Here's how the part is built. I have some questions about the finished solid (model axes, mm). A direction names the side the tool comes from. Coordinates: 2 decimals unless noted, no trailing zeros. Write each loop counter-clockwise with the first axis right and the second up, starting at its lowest first coordinate (ties: lowest second). Pieces come first, ordered by that corner, then holes.
```python
from build123d import *

# Parameters (mm, degrees)
F1_DEPTH = 2


with BuildPart() as f1:
    # F0 (on Top) → F1 (new body)
    with BuildSketch(Plane.XY):
        Polygon((-24.640209, 27.888809), (-21.827112, 25.045134), (-37.467321, 9.5731), (-40.280418, 12.416774), (-60.897057, -7.978181), (56.897057, -7.978181), (36.280418, 12.416774), (33.467321, 9.5731), (17.827112, 25.045134), (20.640209, 27.888809), (5, 43.360843), (5, 53.360843), (-9, 53.360843), (-9, 43.360843), align=None)
        with BuildLine():
            Line((0, 27.021819), (0, 7.021819))
            ThreePointArc((0, 7.021819), (-2, 5.021819), (-4, 7.021819))
            Line((-4, 7.021819), (-4, 27.021819))
            ThreePointArc((-4, 27.021819), (-2, 29.021819), (0, 27.021819))
        make_face(mode=Mode.SUBTRACT)
    extrude(amount=F1_DEPTH)


solid = f1.part
```
1) Imagine slicing it at A-A on z = 0.4. Please give me the cut outline in (x, y).
Values follow:
outline: (-60.9, -7.98) - (56.9, -7.98) - (36.28, 12.42) - (33.47, 9.57) - (17.83, 25.05) - (20.64, 27.89) - (5, 43.36) - (5, 53.36) - (-9, 53.36) - (-9, 43.36) - (-24.64, 27.89) - (-21.83, 25.05) - (-37.47, 9.57) - (-40.28, 12.42) - close; hole (-4, 7.02) arc R2 ccw to (0, 7.02) - (0, 27.02) arc R2 ccw to (-4, 27.02) - close
2) Imagine slicing it at B-B on x = -2. Please give me the cut outline in (y, z).
Values follow:
outline: (-7.98, 0) - (5.02, 0) - (5.02, 2) - (-7.98, 2) - close; (29.02, 0) - (53.36, 0) - (53.36, 2) - (29.02, 2) - close
3) We'd pull the mould along X, two halves only. Please class faces 6 (the face through (-38.854, 10.975, 0.986)), 7 (the face through (-16.711, 35.733, 0.986)), 8 (the face through (5, 48, 1)): pulls with the +X half, pulls with the -X half, needs draft (parallel to the pull), parting line crosses it, or undercut.
Values follow:
face 6: undercut
face 7: pulls with the -X half
face 8: pulls with the +X half
4) I need wall thicknesses on probe 1 along X at (y, z) = (24, 1.25); probe 2 along Y at (x, z) = (19, 1.05); probe 3 along X at (y, z) = (23, 0.15). Which ranges of each line are inside material? Lowest first, please.
Values follow:
probe 1: x = -22.88 to -4, 0 to 18.88
probe 2: y = -7.98 to 23.88, 26.23 to 29.51
probe 3: x = -23.89 to -4, 0 to 19.89
5) On a 3-axis mill with a long thin cutter (end or side, diameter ignored), from which of +Z, -Z, +X, -X, +Y, -Y can I reach the whole of each face in a straight line? I mean faces 1 (the face through (25.76, 17.2, 0.99)), 2 (the face through (19.214, 26.447, 0.986)), 3 (the face through (34.89, 11.01, 0.99)), 4 (the face through (-9, 48, 1)), 5 (the face through (-23.253, 26.487, 0.986)). Say none if no direction works.
Values follow:
face 1: +Z, -Z
face 2: +Z, -Z, +X
face 3: +Z, -Z, +Y
face 4: +Z, -Z, -X, +Y
face 5: +Z, -Z, -X
6) Imagine slicing it at C-C on y = -3. Please give me the cut outline in (x, z).
Values follow:
outline: (-55.86, 0) - (51.86, 0) - (51.86, 2) - (-55.86, 2) - close
7) Will these pins go through, and if not, where does the flat tip stop? pin 1 (1.5 mm diameter, centred on x = -7, y = 12.5, fed in from -Z); pin 2 (1 mm diameter, centred on x = -27.5, y = 22, fed in from -Z).
Values follow:
pin 1: stops at z = 0
pin 2: passes through
8) Imagine slicing it at D-D on x = 13.5. Please give me the cut outline in (y, z).
Values follow:
outline: (-7.98, 0) - (34.95, 0) - (34.95, 2) - (-7.98, 2) - close
